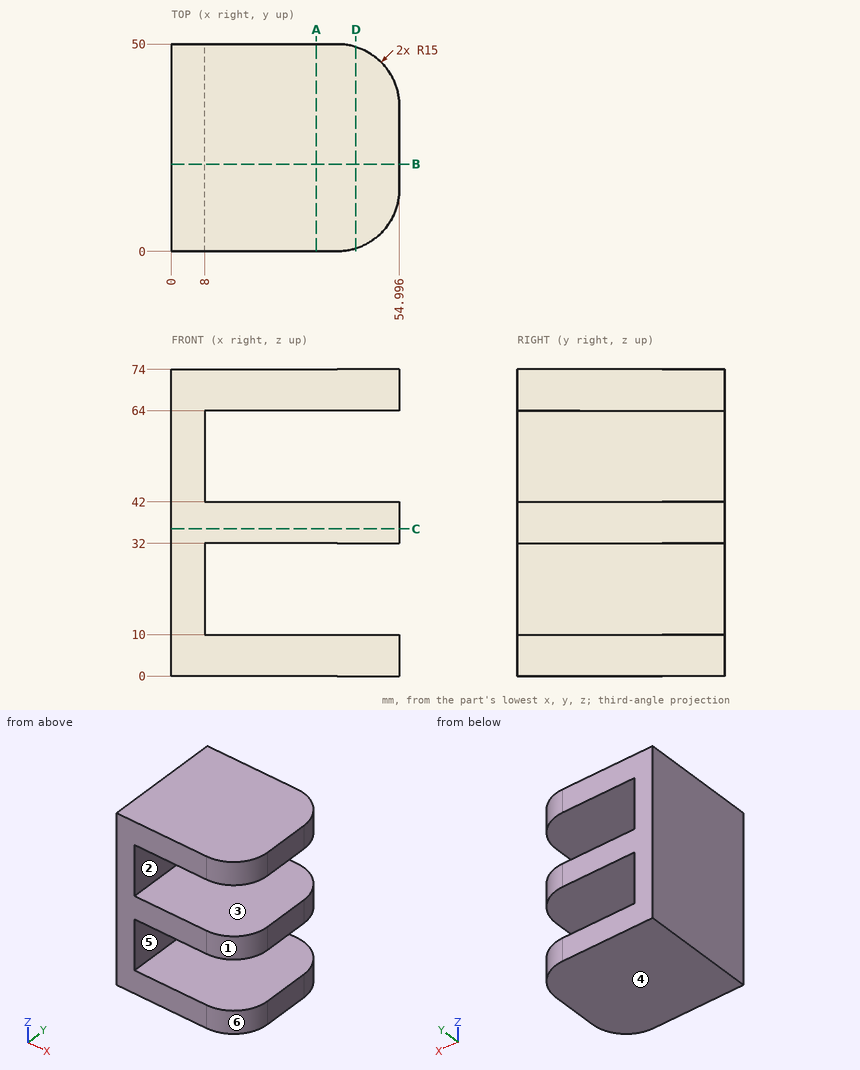
Input: dimensioned drawing with shaded views. Units: mm. Origin: part minimum x, y, z. A direction names the side the tool comes from. Round coordinates to 2 decimals unless told otherwise and drop trailing zeros. Order: outer loops, then holes, each group sorted by start corner. A loop starts at its lowest first (then second) coordinate and runs counter-clockwise, first axis right, second up. Notation, with made-up numbers: M 53.5,35 L 110.5,35 A5 cw 110.5,39 Z; hole C 36.25,65.25 d6. An arc over 180 degrees is marked long. Use one line per item in the form item = value. Start each with the question number.
Q1. Access query for the marked faces 5 and 6. Directions: +Z, -Z, +X, -X, +Y, -Y. A direction counts if a zero-diameter tool reaches every point of the face in a straight line with its end or side. Return the directions, or none.
Q2. Mould query, pull axis Z, two halves, no side actions, for the marked faces 1, 2, 3 and 4. Classes: +Z half, -Z half, draft (parallel to the pull), parting line (faces both ways), or undercut.
Q3. Cut plane B-B (y = 21). Return loops of the section in (x, z), and give its area (3 significant figures).
Q4. Cut plane D-D (x = 44.5). Return loops of the section in (y, z).
Q5. Cut plane A-A (x = 35). Return loops of the section in (y, z).
Q6. Material intervals for line 1 (Z direction, x = 44, y = 11); line 2 (X direction, y = 20, z = 49); line 3 (Y direction, x = 44, z = 35), sorted ascending. Write a range as [from, to].
Q7. Pin query (flat end, axial travel): pin 1 Ø1.5 at (y, z) = (6, 18.5) entering from +X. Return the tip coordinate at first contact, or that it passes through.
Q8. Cut plane C-C (z = 35.5). Return loops of the section in (x, y).
Geometry results:
q1.face_5 = +X, +Y, -Y
q1.face_6 = +Z, -Z, +X, -Y
q2.face_1 = draft
q2.face_2 = undercut
q2.face_3 = undercut
q2.face_4 = -Z half
q3.outline = M 0,0 L 55,0 L 55,10 L 8,10 L 8,32 L 55,32 L 55,42 L 8,42 L 8,64 L 55,64 L 55,74 L 0,74 Z
q3.area = 2,000 mm^2
q4.outline = M 0.69,0 L 49.31,0 L 49.31,10 L 0.69,10 Z; M 0.69,32 L 49.31,32 L 49.31,42 L 0.69,42 Z; M 0.69,64 L 49.31,64 L 49.31,74 L 0.69,74 Z
q5.outline = M 0,0 L 50,0 L 50,10 L 0,10 Z; M 0,32 L 50,32 L 50,42 L 0,42 Z; M 0,64 L 50,64 L 50,74 L 0,74 Z
q6.line_1 = [0, 10], [32, 42], [64, 74]
q6.line_2 = [0, 8]
q6.line_3 = [0.54, 49.46]
q7.pin_1 = 8
q8.outline = M 0,0 L 40,0 A15 ccw 55,15 L 55,35 A15 ccw 40,50 L 0,50 Z
